Verification items for the finished model (mm, model axes). A direction names the side the tool comes from. Coordinates: 2 decimals unless noted, no trailing zeros. Loops run counter-clockwise (first coordinate to the right, second up) from the corner with the lowest first, then second, coordinate; pieces in that order, holes last. Notation, with made-up numbers: (65, -18.75) -> (105, -18.75) arc R26 ccw to (105, 10.25) -> close; hole circle Ø10 at (-6.75, 17.25). An arc over 180 degrees is marked (long way). Write item = value, one per line.
```python
from build123d import *

# Parameters (mm, degrees)
SKETCH1_W           = 7
SKETCH1_H           = 7
BOSS_EXTRUDE1_DEPTH = 3
CUT_EXTRUDE1_DEPTH  = 7
CUT_EXTRUDE2_DEPTH  = 11
SKETCH4_R           = 1.8
CUT_EXTRUDE3_DEPTH  = 0.8
CUT_EXTRUDE4_DEPTH  = 0.4


with BuildPart() as part:
    # Sketch1 → Boss-Extrude1 (new body)
    with BuildSketch(Plane(origin=(0, 0, 0), x_dir=(1, 0, 0), z_dir=(0, 1, 0))):
        with Locations((3.5, 3.5)):
            Rectangle(SKETCH1_W, SKETCH1_H)
    extrude(amount=BOSS_EXTRUDE1_DEPTH)

    # Sketch2 → Cut-Extrude1 (cut)
    with BuildSketch(Plane.XY):
        Polygon((0, 0), (0.7, 3), (0, 3), align=None)
        Polygon((7, 0), (6.3, 3), (7, 3), align=None)
    extrude(amount=-CUT_EXTRUDE1_DEPTH, mode=Mode.SUBTRACT)

    # Sketch3 → Cut-Extrude2 (cut)
    with BuildSketch(Plane(origin=(0, 0, 0), x_dir=(0, 0, -1), z_dir=(1, 0, 0))):
        Polygon((0, 0), (0.7, 3), (0, 3), align=None)
        Polygon((7, 3), (6.3, 3), (7, 0), align=None)
    extrude(amount=CUT_EXTRUDE2_DEPTH, mode=Mode.SUBTRACT)

    # Sketch4 → Cut-Extrude3 (cut)
    with BuildSketch(Plane.XZ):
        with Locations(Location((3.5, -3.5, 0), (0, 0, 270))):
            Circle(SKETCH4_R)
    extrude(amount=-CUT_EXTRUDE3_DEPTH, mode=Mode.SUBTRACT)

    # Sketch5 → Cut-Extrude4 (cut)
    with BuildSketch(Plane(origin=(0, 3, 0), x_dir=(1, 0, 0), z_dir=(0, 1, 0))):
        Polygon((2.253196063, 1.786270222), (2.253196063, 5.286270222), (2.926272986, 5.286270222), (2.926272986, 2.369603555), (4.721144781, 2.369603555), (4.721144781, 1.786270222), align=None)
    extrude(amount=-CUT_EXTRUDE4_DEPTH, mode=Mode.SUBTRACT)


solid = part.part
```
1) Tool access check on faces 4 (the face through (0.345, 1.479, -3.451)), 5 (the face through (4.041, 0.394, -5.217)). Record the directions out of +Z, -Z, +X, -X, +Y, -Y that give a thin tool (end or side, any length) a straight path to the whole face; none if there is none.
Ans:
face_4 = +Z, -Z, -X, +Y
face_5 = -Y
2) Release check for a two-part mould opening along X. For faces 1 (the face through (6.655, 1.479, -3.451)), 2 (the face through (3.451, 1.521, -6.645)), 3 (the face through (2.76, 2.6, -3.16)) record: pulls with the +X half, pulls with the -X half, needs draft (parallel to the pull), parting line crosses it, or undercut.
Ans:
face_1 = pulls with the +X half
face_2 = needs draft
face_3 = undercut
3) Sectioned sample at B-B, the plane x = 3.5. Record the cut outline in (y, z), plus the area to 3 significant figures.
Ans:
outline = (0, -7) -> (3, -6.3) -> (3, -2.37) -> (2.6, -2.37) -> (2.6, -1.79) -> (3, -1.79) -> (3, -0.7) -> (0, 0) -> (0, -1.7) -> (0.8, -1.7) -> (0.8, -5.3) -> (0, -5.3) -> close
area = 15.8 mm2
4) Sectioned sample at C-C, the plane z = -3.5. Record the cut outline in (x, y), plus the area to 3 significant figures.
Ans:
outline = (0, 0) -> (1.7, 0) -> (1.7, 0.8) -> (5.3, 0.8) -> (5.3, 0) -> (7, 0) -> (6.3, 3) -> (2.93, 3) -> (2.93, 2.6) -> (2.25, 2.6) -> (2.25, 3) -> (0.7, 3) -> close
area = 15.8 mm2
5) Material ranges on line 1 (Y direction, x = 4, z = -5); line 2 (Z direction, x = 2.25, y = 0.4); line 3 (X direction, y = 2.95, z = -2), recorded low to high.
Ans:
line_1 = 0.8 to 3
line_2 = -6.91 to -4.8, -2.2 to -0.09
line_3 = 0.69 to 2.25, 4.72 to 6.31
6) Sectioned sample at D-D, the plane y = 2.1. Record the cut outline in (x, z).
Ans:
outline = (0.49, -6.51) -> (6.51, -6.51) -> (6.51, -0.49) -> (0.49, -0.49) -> close
7) Depth check by flat-ended pin: pin 1 Ø1 at (x, y) = (4.5, 1) entering from +Z; pin 2 Ø1.1 at (x, z) = (4, -4) entering from -Y; pin 3 Ø1 at (y, z) = (1.5, -1.5) entering from +X. Enter the tip coordinate at first touch or a pass-through.
Ans:
pin_1 = -0.12
pin_2 = 0.8
pin_3 = 6.77
8) Sectioned sample at A-A, the plane y = 0.3. Record the cut outline in (x, z).
Ans:
outline = (0.07, -6.93) -> (6.93, -6.93) -> (6.93, -0.07) -> (0.07, -0.07) -> close; hole circle Ø3.6 at (3.5, -3.5)
